For this review, use the dimensioned drawing (mm, ordinates from the lowest corner) and the shaded views. A direction names the side the tool comes from. Round coordinates to 2 decimals unless told otherwise and drop trailing zeros. Loops run counter-clockwise (first coordinate to the right, second up) from the corner with the lowest first, then second, coordinate; pieces in that order, holes last. Notation, with made-up numbers: (87, -31.75) -> (98, -31.75) arc R29 ccw to (98, -1.75) -> close; hole circle Ø1 at (47, 66). An arc over 180 degrees is marked (long way). Write each question's results on one line, items separated by ' | '.
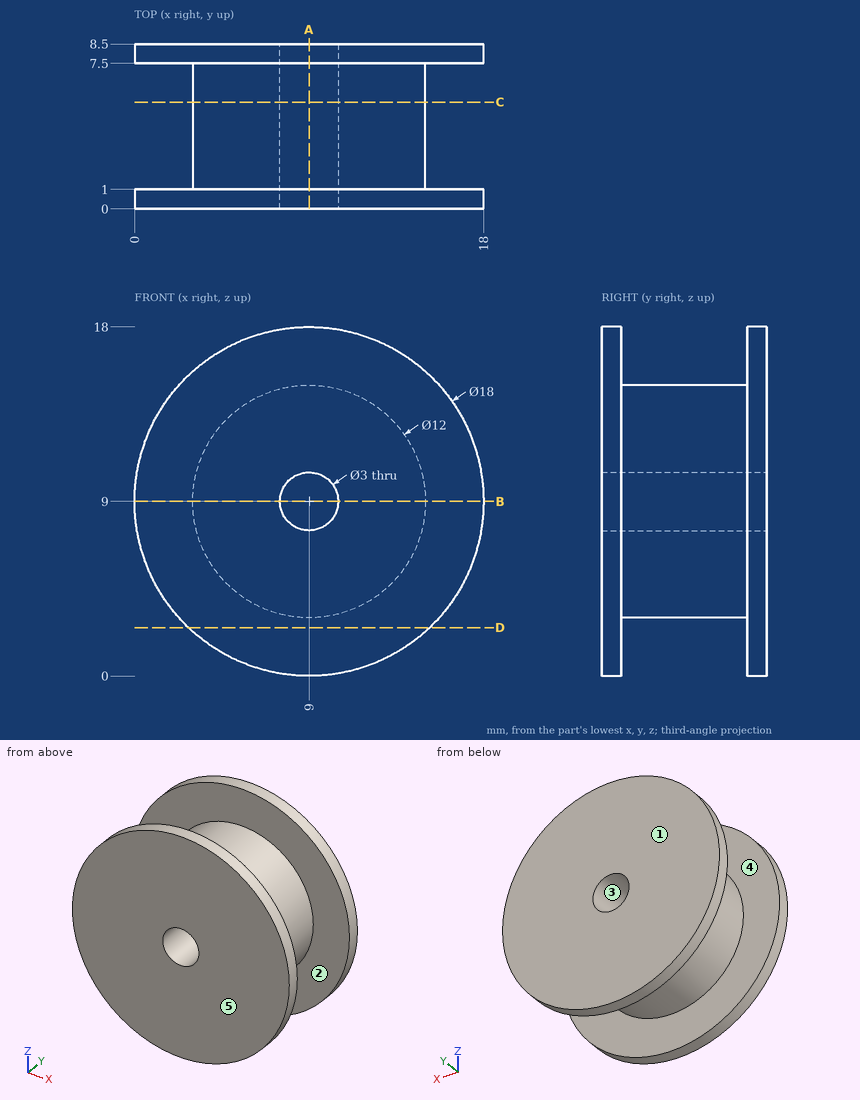
1. Consider section A-A (x = 9). State the section outline as (y, z) points, plus the area to 3 significant figures.
Values found:
outline: (0, 0) -> (1, 0) -> (1, 3) -> (7.5, 3) -> (7.5, 0) -> (8.5, 0) -> (8.5, 7.5) -> (0, 7.5) -> close; (0, 10.5) -> (8.5, 10.5) -> (8.5, 18) -> (7.5, 18) -> (7.5, 15) -> (1, 15) -> (1, 18) -> (0, 18) -> close | area: 88.5 mm2
2. Draft analysis for pull direction Y (two halves, no side actions). For the marked faces 3, 4 and 5, state which applies: released by +Y, released by -Y, zero draft, split by the parting line, or undercut.
Values found:
face 3: zero draft | face 4: undercut | face 5: released by -Y
3. To check wall thickness, follow probe 1 along Z at (x, y) = (9, 6.5); probe 2 along Y at (x, z) = (4.5, 15). State the ranges of each line that lie inside material, in increasing order.
Values found:
probe 1: z = 3 to 7.5, 10.5 to 15 | probe 2: y = 0 to 1, 7.5 to 8.5
4. For pin 1 (1 mm diameter, centred on x = 15, y = 4.5, fed in from +Z); pin 2 (2 mm diameter, centred on y = 7, z = 15.5, fed in from -X); pin 3 (3 mm diameter, centred on y = 2, z = 2, fed in from +X), all flat-tipped, find the tip position at first contact; note any pin that passes through.
Values found:
pin 1: stops at z = 11.4 | pin 2: stops at x = 1.98 | pin 3: stops at x = 15.81
5. Consider section D-D (z = 2.5). State the section outline as (x, y) points.
Values found:
outline: (2.78, 0) -> (15.22, 0) -> (15.22, 1) -> (2.78, 1) -> close; (2.78, 7.5) -> (15.22, 7.5) -> (15.22, 8.5) -> (2.78, 8.5) -> close
6. Consider section B-B (z = 9). State the section outline as (x, y) points, plus the area to 3 significant figures.
Values found:
outline: (0, 0) -> (7.5, 0) -> (7.5, 8.5) -> (0, 8.5) -> (0, 7.5) -> (3, 7.5) -> (3, 1) -> (0, 1) -> close; (10.5, 0) -> (18, 0) -> (18, 1) -> (15, 1) -> (15, 7.5) -> (18, 7.5) -> (18, 8.5) -> (10.5, 8.5) -> close | area: 88.5 mm2
7. Tool access review of the marked faces 1 and 2: name each direction out of +Z, -Z, +X, -X, +Y, -Y from which nothing blocks a thin tool from reaching the whole face with its end or side.
Values found:
face 1: +Z, -Z, +X, -X, +Y | face 2: none
8. Consider section C-C (y = 5.5). State the section outline as (x, z) points, plus the area to 3 significant figures.
Values found:
outline: circle Ø12 at (9, 9); hole circle Ø3 at (9, 9) | area: 106 mm2
